Input: dimensioned drawing with shaded views. Units: mm. Origin: part minimum x, y, z. A direction names the side the tool comes from. Give positions to 0.01 mm unless a question says otherwise; leave off trailing zeros. Write each loop counter-clockwise with the first axis right and the second up, starting at its lowest first coordinate (ties: lowest second). Pieces come first, ordered by that corner, then holes. Notation, with made-up numbers: (7, 66.25) -> (57, 66.25) arc R24 ccw to (57, 102.25) -> close; hole circle Ø5 at (76, 39). An arc over 180 degrees is marked (long way). Answer as a JSON object with one key per item and string values. Group by question number.
(1) Contact query for flat-ended pins moving along their axis: pin 1 Ø5 at (x, y) = (12, 22.5) entering from +Z; pin 2 Ø3.5 at (x, y) = (17.5, 26.25) entering from +Z; pin 3 Ø10 at (y, z) = (17.5, 49.5) entering from +X. Output: stop coordinate, or through.
(2) Section query A-A on x = 17.5. Output: boundary loops of the cut face in (y, z), plus the area to 3 significant figures.
(3) Set-up query: the marked faces 1 and 2. Return all of +Z, -Z, +X, -X, +Y, -Y with unobstructed straight access to the full face (end or side cutting, diameter ignored); none if empty.
(4) Section query C-C on y = 3.5. Output: boundary loops of the cut face in (x, z).
(5) Material intervals for probe 1 along Y at (x, z) = (17.5, 5.75); probe 2 along Z at (x, y) = (5.5, 17.5); probe 3 along X at (y, z) = (8.75, 6), sorted ascending.
(6) Section query B-B on x = 5.25. Output: boundary loops of the cut face in (y, z).
(7) Section query D-D on y = 26.25. Output: boundary loops of the cut face in (x, z).
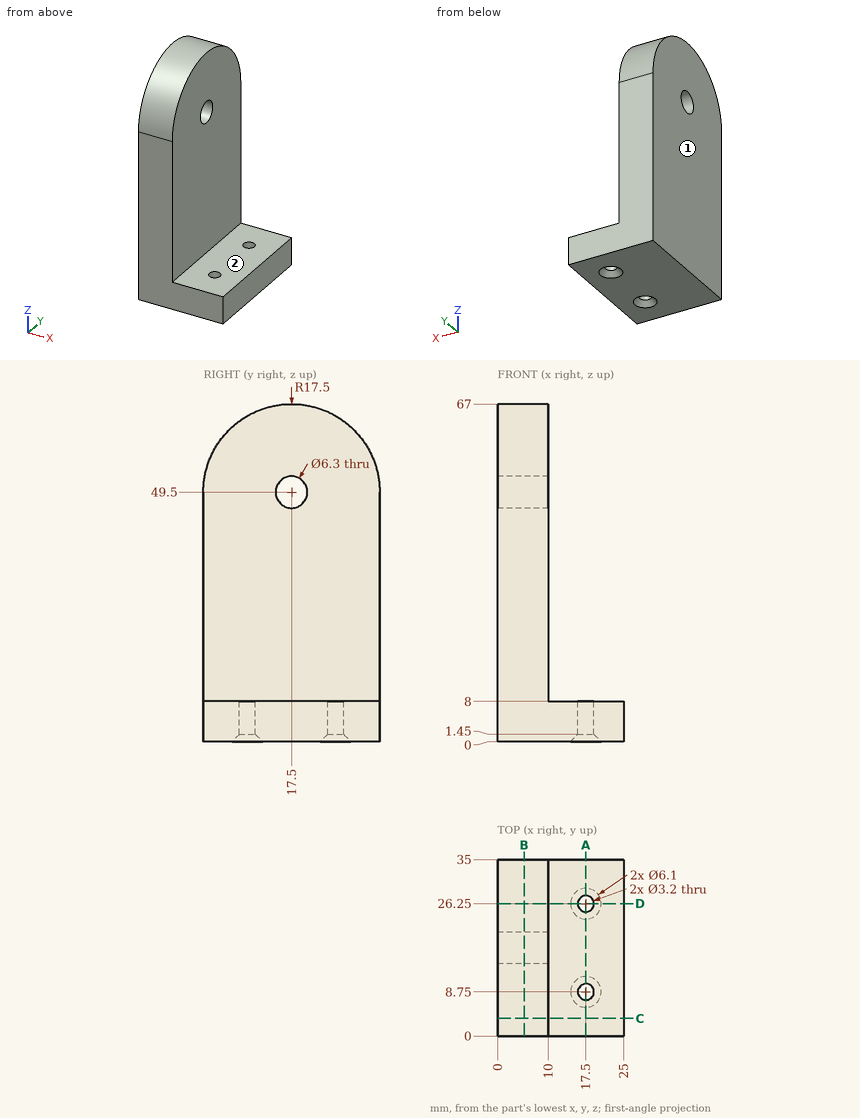
Answer list:
{
 "1": {"pin 1": "z = 66.65", "pin 2": "z = 8", "pin 3": "x = 10"},
 "2": {"outline": "(0, 0) -> (5.7, 0) -> (7.15, 1.45) -> (7.15, 8) -> (0, 8) -> close; (10.35, 1.45) -> (11.8, 0) -> (23.2, 0) -> (24.65, 1.45) -> (24.65, 8) -> (10.35, 8) -> close; (27.85, 1.45) -> (29.3, 0) -> (35, 0) -> (35, 8) -> (27.85, 8) -> close", "area": "225 mm2"},
 "3": {"face 1": "+Z, -Z, -X, +Y, -Y", "face 2": "+Z, +X, +Y, -Y"},
 "4": {"outline": "(0, 0) -> (25, 0) -> (25, 8) -> (10, 8) -> (10, 60) -> (0, 60) -> close"},
 "5": {"probe 1": "0 to 7.15, 10.35 to 24.65, 27.85 to 35", "probe 2": "0 to 46.35, 52.65 to 67", "probe 3": "0 to 15.9, 19.1 to 25"},
 "6": {"outline": "(0, 0) -> (35, 0) -> (35, 49.5) arc R17.5 ccw to (0, 49.5) -> close; hole circle Ø6.3 at (17.5, 49.5)"},
 "7": {"outline": "(0, 0) -> (14.45, 0) -> (15.9, 1.45) -> (15.9, 8) -> (10, 8) -> (10, 64.66) -> (0, 64.66) -> close; (19.1, 1.45) -> (20.55, 0) -> (25, 0) -> (25, 8) -> (19.1, 8) -> close"}
}
